The listing builds one solid part. Answer for the finished solid, in the listing's coordinates (mm). Round coordinates to 2 decimals unless told otherwise and drop trailing zeros. Write each loop counter-clockwise with the first axis right and the second up, starting at its lowest first coordinate (ties: lowest second). Pieces come first, ordered by that corner, then holes.
(1) A cutting plane is placed at A-A, the plane y = 43. Give the vertices of the cut face in (x, z), and give its area (3 significant figures).
(2) Find the intervals of material crossed by probe 1 along X at (y, z) = (-76.5, 2.9); probe 2 along Y at (x, z) = (-131.5, 3.2); probe 3 along X at (y, z) = (50.5, 0.6), in increasing order.
(3) A cutting plane is placed at C-C, the plane x = 118. Give the vertices of the cut face in (y, z).
(4) Each of these flat-tipped pins is pushed along its axis until it touches: pin 1 Ø2 at (x, y) = (0, -76.5) entering from +Z; pin 2 Ø1.3 at (y, z) = (66, 2.5) entering from +X; pin 3 Ø2 at (x, z) = (5, 2.5) entering from +Y; pin 4 Ø1.3 at (y, z) = (56, 1.5) entering from -X. Where does it stop, or does it pass through?
(5) A cutting plane is placed at B-B, the plane z = 1.15. Give the vertices of the cut face in (x, y) (3 decimals).
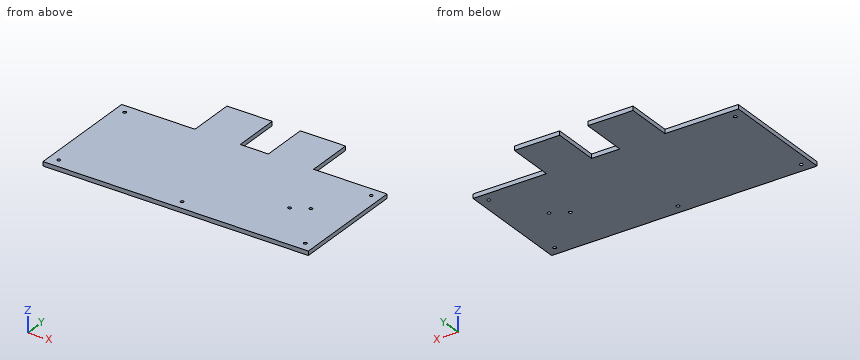
from build123d import *

# Parameters (mm, degrees)
SKETCH1_W           = 283
SKETCH1_H           = 173
SKETCH1_R           = 1.75
BOSS_EXTRUDE1_DEPTH = 4.5
CUT_EXTRUDE1_REACH  = 6.5
SKETCH2_W           = 78.25
SKETCH2_H           = 50
SKETCH2_W_2         = 30
SKETCH3_R           = 1.75
CUT_EXTRUDE2_DEPTH  = 10
CUT_EXTRUDE4_REACH  = 6.5
SKETCH5_R           = 1.75


with BuildPart() as part:
    # Sketch1 → Boss-Extrude1 (new body)
    with BuildSketch(Plane.XY):
        Rectangle(SKETCH1_W, SKETCH1_H)
        with Locations((-131.5, 76.5)):
            Circle(SKETCH1_R, mode=Mode.SUBTRACT)
        with Locations((-131.5, 76.5)):
            Circle(SKETCH1_R)
    extrude(amount=BOSS_EXTRUDE1_DEPTH)

    # Sketch2 → Cut-Extrude1 (cut, up to next)
    with BuildSketch(Plane.XY.offset(4.5), mode=Mode.PRIVATE) as cut_extrude1_sk1:
        with Locations((102.375, 61.5)):
            Rectangle(SKETCH2_W, SKETCH2_H)
    cut_extrude1_tool1 = extrude(cut_extrude1_sk1.sketch, amount=-CUT_EXTRUDE1_REACH, mode=Mode.PRIVATE) & part.part
    add(cut_extrude1_tool1.solids().sort_by_distance((102.375, 61.5, 4.5))[0], mode=Mode.SUBTRACT)
    # Sketch2 → Cut-Extrude1 (cut, up to next)
    with BuildSketch(Plane.XY.offset(4.5), mode=Mode.PRIVATE) as cut_extrude1_sk2:
        with Locations((-102.375, 61.5)):
            Rectangle(SKETCH2_W, SKETCH2_H)
    cut_extrude1_tool2 = extrude(cut_extrude1_sk2.sketch, amount=-CUT_EXTRUDE1_REACH, mode=Mode.PRIVATE) & part.part
    add(cut_extrude1_tool2.solids().sort_by_distance((-102.375, 61.5, 4.5))[0], mode=Mode.SUBTRACT)
    # Sketch2 → Cut-Extrude1 (cut, up to next)
    with BuildSketch(Plane.XY.offset(4.5), mode=Mode.PRIVATE) as cut_extrude1_sk3:
        with Locations((0, 61.5)):
            Rectangle(SKETCH2_W_2, SKETCH2_H)
    cut_extrude1_tool3 = extrude(cut_extrude1_sk3.sketch, amount=-CUT_EXTRUDE1_REACH, mode=Mode.PRIVATE) & part.part
    add(cut_extrude1_tool3.solids().sort_by_distance((0, 61.5, 4.5))[0], mode=Mode.SUBTRACT)

    # Sketch3 → Cut-Extrude2 (cut)
    with BuildSketch(Plane.XY.offset(4.5)):
        with Locations((-131.5, -76.5)):
            Circle(SKETCH3_R)
        with Locations((131.5, -76.5)):
            Circle(SKETCH3_R)
        with Locations((131.5, 26.5)):
            Circle(SKETCH3_R)
        with Locations((-131.5, 26.5)):
            Circle(SKETCH3_R)
        with Locations((0, -76.5)):
            Circle(SKETCH3_R)
    extrude(amount=-CUT_EXTRUDE2_DEPTH, mode=Mode.SUBTRACT)

    # Sketch5 → Cut-Extrude4 (cut, up to next)
    with BuildSketch(Plane.XY.offset(4.5), mode=Mode.PRIVATE) as cut_extrude4_sk1:
        with Locations((84.512023679, -32.2)):
            Circle(SKETCH5_R)
    cut_extrude4_tool1 = extrude(cut_extrude4_sk1.sketch, amount=-CUT_EXTRUDE4_REACH, mode=Mode.PRIVATE) & part.part
    add(cut_extrude4_tool1.solids().sort_by_distance((84.512024, -32.2, 4.5))[0], mode=Mode.SUBTRACT)
    # Sketch5 → Cut-Extrude4 (cut, up to next)
    with BuildSketch(Plane.XY.offset(4.5), mode=Mode.PRIVATE) as cut_extrude4_sk2:
        with Locations((100.75, -22.825)):
            Circle(SKETCH5_R)
    cut_extrude4_tool2 = extrude(cut_extrude4_sk2.sketch, amount=-CUT_EXTRUDE4_REACH, mode=Mode.PRIVATE) & part.part
    add(cut_extrude4_tool2.solids().sort_by_distance((100.75, -22.825, 4.5))[0], mode=Mode.SUBTRACT)


solid = part.part
Solutions:
1. outline: (-63.25, 0) - (-15, 0) - (-15, 4.5) - (-63.25, 4.5) - close; (15, 0) - (63.25, 0) - (63.25, 4.5) - (15, 4.5) - close
1. area: 434 mm2
2. probe 1: x = -141.5 to -133.25, -129.75 to -1.75, 1.75 to 129.75, 133.25 to 141.5
2. probe 2: y = -86.5 to -78.25, -74.75 to 24.75, 28.25 to 36.5
2. probe 3: x = -63.25 to -15, 15 to 63.25
3. outline: (-86.5, 0) - (36.5, 0) - (36.5, 4.5) - (-86.5, 4.5) - close
4. pin 1: passes through
4. pin 2: stops at x = 63.25
4. pin 3: stops at y = 36.5
4. pin 4: stops at x = -63.25
5. outline: (-141.5, -86.5) - (141.5, -86.5) - (141.5, 36.5) - (63.25, 36.5) - (63.25, 86.5) - (15, 86.5) - (15, 36.5) - (-15, 36.5) - (-15, 86.5) - (-63.25, 86.5) - (-63.25, 36.5) - (-141.5, 36.5) - close; hole circle Ø3.5 at (-131.5, -76.5); hole circle Ø3.5 at (-131.5, 26.5); hole circle Ø3.5 at (0, -76.5); hole circle Ø3.5 at (84.512, -32.2); hole circle Ø3.5 at (100.75, -22.825); hole circle Ø3.5 at (131.5, -76.5); hole circle Ø3.5 at (131.5, 26.5)
